```python
from build123d import *

# Parameters (mm, degrees)
SKETCH11_R               = 2.354570308
MEMBER_10_1012_S_1_DEPTH = 50.8


with BuildPart() as part:
    # Sketch11 → Member 10 1012-S_1 (new body)
    with BuildSketch(Plane(origin=(0, 0, 0), x_dir=(-1, 0, 0), z_dir=(0, 1, 0))):
        with BuildLine():
            Line((24.2951, 0), (16.9672, 0))
            ThreePointArc((16.9672, 0), (16.24877951, -0.29757951), (15.9512, -1.016))
            Line((15.9512, -1.016), (15.9512, -1.1938))
            ThreePointArc((15.9512, -1.1938), (16.24877951, -1.91222049), (16.9672, -2.2098))
            Line((16.9672, -2.2098), (19.174794456, -2.2098))
            ThreePointArc((19.174794456, -2.2098), (20.113456061, -2.836993633), (19.893214945, -3.94422049))
            Line((19.893214945, -3.94422049), (15.930814945, -7.90662049))
            ThreePointArc((15.930814945, -7.90662049), (15.601200823, -8.126861605), (15.212394456, -8.2042))
            Line((15.212394456, -8.2042), (10.187605544, -8.2042))
            ThreePointArc((10.187605544, -8.2042), (9.798799177, -8.126861605), (9.469185055, -7.90662049))
            Line((9.469185055, -7.90662049), (5.506785055, -3.94422049))
            ThreePointArc((5.506785055, -3.94422049), (5.286543939, -2.836993633), (6.225205544, -2.2098))
            Line((6.225205544, -2.2098), (8.4328, -2.2098))
            ThreePointArc((8.4328, -2.2098), (9.15122049, -1.91222049), (9.4488, -1.1938))
            Line((9.4488, -1.1938), (9.4488, -1.016))
            ThreePointArc((9.4488, -1.016), (9.15122049, -0.29757951), (8.4328, 0))
            Line((8.4328, 0), (1.1049, 0))
            ThreePointArc((1.1049, 0), (0.323617717, -0.323617717), (0, -1.1049))
            Line((0, -1.1049), (0, -8.4328))
            ThreePointArc((0, -8.4328), (0.29757951, -9.15122049), (1.016, -9.4488))
            Line((1.016, -9.4488), (1.1938, -9.4488))
            ThreePointArc((1.1938, -9.4488), (1.91222049, -9.15122049), (2.2098, -8.4328))
            Line((2.2098, -8.4328), (2.2098, -6.225205544))
            ThreePointArc((2.2098, -6.225205544), (2.836993633, -5.286543939), (3.94422049, -5.506785055))
            Line((3.94422049, -5.506785055), (7.90662049, -9.469185055))
            ThreePointArc((7.90662049, -9.469185055), (8.126861605, -9.798799177), (8.2042, -10.187605544))
            Line((8.2042, -10.187605544), (8.2042, -15.212394456))
            ThreePointArc((8.2042, -15.212394456), (8.126861605, -15.601200823), (7.90662049, -15.930814945))
            Line((7.90662049, -15.930814945), (3.94422049, -19.893214945))
            ThreePointArc((3.94422049, -19.893214945), (2.836993633, -20.113456061), (2.2098, -19.174794456))
            Line((2.2098, -19.174794456), (2.2098, -16.9672))
            ThreePointArc((2.2098, -16.9672), (1.91222049, -16.24877951), (1.1938, -15.9512))
            Line((1.1938, -15.9512), (1.016, -15.9512))
            ThreePointArc((1.016, -15.9512), (0.29757951, -16.24877951), (0, -16.9672))
            Line((0, -16.9672), (0, -24.2951))
            ThreePointArc((0, -24.2951), (0.323617717, -25.076382283), (1.1049, -25.4))
            Line((1.1049, -25.4), (6.35, -25.4))
            ThreePointArc((6.35, -25.4), (19.820384182, -19.820384182), (25.4, -6.35))
            Line((25.4, -6.35), (25.4, -1.1049))
            ThreePointArc((25.4, -1.1049), (25.076382283, -0.323617717), (24.2951, 0))
        make_face()
        with Locations((12.7, -12.7)):
            Circle(SKETCH11_R, mode=Mode.SUBTRACT)
    extrude(amount=MEMBER_10_1012_S_1_DEPTH)


solid = part.part
```
Can you work these out from the model? Positions are in its coordinate system, mm. A direction names the side the tool comes from. Round coordinates to 2 decimals unless told otherwise and drop trailing zeros. Loops run counter-clockwise (first coordinate to the right, second up) from the corner with the lowest first, then second, coordinate; pieces in that order, holes last.
Item 1: Will these pins go through, and if not, where does the flat tip stop? pin 1 Ø6 at (x, y) = (-16, 43.5) entering from -Z; pin 2 Ø6 at (x, y) = (-13.5, 43.5) entering from -Z; pin 3 Ø5.5 at (y, z) = (35, -13) entering from +X.
Item 2: Suppose I cut it at B-B, the plane z = -12.7. Write out the boundary of the cut face in (x, y), then the cut area to 3 significant figures.
Item 3: Please list where these lines run through material, in increasing order: L1, parallel to Z at x = -6.25, y = 38.5; L2, parallel to Z at x = -7, y = 21.5; L3, parallel to Z at x = -12.7, y = 28.5.
Item 4: Which directions (+Z, -Z, +X, -X, +Y, -Y) give clear straight access to the entire face, cutting with the end or side of a thin tool? Please do faces 4 (the cylindrical face through (-0.32, 25.04, -25.07)), 5 (the cylindrical face through (-5.28, 25.04, -2.85)), 6 (the cylindrical face through (-0.29, 25.044, -9.143)).
Item 5: If we mould it in two halves opening along Z, with no side actions, what happens to faces 1 (the cylindrical face through (-19.67, 25.04, -19.97)), 2 (the cylindrical face through (-9.159, 25.044, -0.306)), 3 (the cylindrical face through (-9.143, 25.044, -1.92))? For each: +Z half, -Z half, draft (parallel to the pull), parting line (faces both ways), or undercut.
Item 6: Suppose I cut it at A-A, the plane x = -14.5. Write out the boundary of the cut face in (y, z).
Item 7: Suppose I cut it at C-C, the plane x = -23.5. Write out the boundary of the cut face in (y, z).
Reported:
1. pin 1: stops at z = -24.2
1. pin 2: stops at z = -24.94
1. pin 3: stops at x = -8.05
2. outline: (-24.31, 0) - (-15.05, 0) - (-15.05, 50.8) - (-24.31, 50.8) - close; (-10.35, 0) - (-8.2, 0) - (-8.2, 50.8) - (-10.35, 50.8) - close
2. area: 579 mm2
3. L1: z = -25.4 to -17.59, -7.81 to -4.69, -2.21 to 0
3. L2: z = -25.39 to -16.84, -8.56 to -5.44, -2.21 to 0
3. L3: z = -24.31 to -15.05, -10.35 to -8.2
4. face 4: -Z, +X, +Y, -Y
4. face 5: +Y, -Y
4. face 6: +X, +Y, -Y
5. face 1: -Z half
5. face 2: +Z half
5. face 3: undercut
6. outline: (0, -23.57) - (50.8, -23.57) - (50.8, -14.22) - (0, -14.22) - close; (0, -11.18) - (50.8, -11.18) - (50.8, -8.2) - (0, -8.2) - close
7. outline: (0, -14.64) - (50.8, -14.64) - (50.8, 0) - (0, 0) - close
